Build history of the part. All positions in model axes, mm. Face numbers are marked on the shaded views. A direction names the side the tool comes from. Give positions to 0.01 mm unless a question says otherwise; leave off trailing zeros. Loops run counter-clockwise (first coordinate to the right, second up) from the corner with the lowest first, then second, coordinate; pieces in that order, holes last. Notation, with made-up numbers: (58, 70) -> (83, 70) arc R24 ccw to (83, 95) -> close; hole circle Ø1 at (6, -1). An arc over 180 degrees is marked (long way). One line per question, with ' | ' between items. Start each with the question number.
(1) 3-axis set-ups, long thin cutter, end or side, ignore diameter. For the marked faces 5, 6, 7 and 8: which of +Z, -Z, +X, -X, +Y, -Y reach the whole face in a straight line?
(2) Slice it at C-C, the plane z = 27. Write the cut outline in (x, y), then the cut area to 3 significant figures.
(3) Mould opens along X. For the marked faces 1, 2, 3 and 4 say: pulls with the +X half, pulls with the -X half, needs draft (parallel to the pull), parting line crosses it, or undercut.
(4) Slice it at A-A, the plane x = 26. Write the cut outline in (y, z), then the cut area to 3 significant figures.
(5) Slice it at B-B, the plane y = 44.5. Write the cut outline in (x, z), then the cut area to 3 significant figures.
(6) Slice it at D-D, the plane z = 14. Write the cut outline in (x, y), then the cut area to 3 significant figures.
(7) Flat gauge pins, fed straight in: pin 1 Ø2.5 at (x, z) = (25, 13.5) entering from -Y; pin 2 Ø1.6 at (x, z) = (14, 16) entering from -Y; pin 3 Ø13 at (x, z) = (36, 28) entering from +Y; pin 4 Ø1 at (x, y) = (10.5, 16.5) entering from +Z. Where does each tip first touch, or does it go through?
(8) Drill centre lines: L1, parallel to Y at x = 9, z = 13.25; L2, parallel to Y at x = 10.5, z = 14.75; L3, parallel to Y at x = 25, z = 25.5. Where is each one in solid material? Low to high. Write a range as from..to.
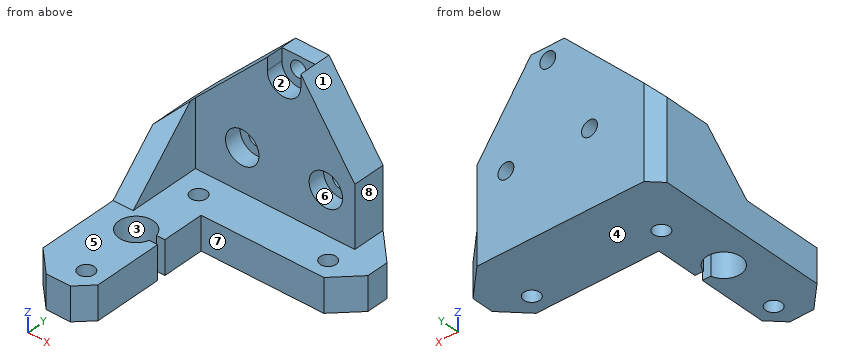
```python
from build123d import *

# Parameters (mm, degrees)
SKETCH_R        = 1.9
SKETCH_R_2      = 4.1
PAD_DEPTH       = 8
PAD001_DEPTH    = 33
SKETCH002_R     = 1.9
POCKET_DEPTH    = 7.801
POCKET001_DEPTH = 5
POCKET002_DEPTH = 50.001
CHAMFER_SIZE    = 3
SKETCH005_R     = 4
POCKET003_DEPTH = 4
SKETCH006_W     = 2.5
SKETCH006_H     = 2
POCKET004_DEPTH = 8.001


with BuildPart() as part:
    # Sketch → Pad (new body)
    with BuildSketch(Plane.XY.offset(10)):
        Polygon((0, 50), (0, 5.656854), (5.656854, 0), (11.464466, 0), (15, 3.535534), (15, 32), (44.343146, 32), (50, 37.656854), (50, 42.928932), (42.928932, 50), align=None)
        with Locations((41.5, 36.5)):
            Circle(SKETCH_R, mode=Mode.SUBTRACT)
        with Locations((10.5, 36.5)):
            Circle(SKETCH_R, mode=Mode.SUBTRACT)
        with Locations((10.5, 5.5)):
            Circle(SKETCH_R, mode=Mode.SUBTRACT)
        with Locations((9, 21)):
            Circle(SKETCH_R_2, mode=Mode.SUBTRACT)
    extrude(amount=PAD_DEPTH)

    # Sketch001 → Pad001 (new body)
    with BuildSketch(Plane.XY.offset(18)):
        Polygon((42.928932, 50), (0, 50), (0, 25), (4.8, 25), (4.8, 42.2), (42.928932, 42.2), align=None)
    extrude(amount=PAD001_DEPTH)

    # Sketch002 → Pocket (cut, through all)
    with BuildSketch(Plane(origin=(0, 42.2, 10), x_dir=(1, 0, 0), z_dir=(0, -1, 0))):
        with Locations((26, 38)):
            Circle(SKETCH002_R)
        with Locations((16, 18)):
            Circle(SKETCH002_R)
        with Locations((36, 18)):
            Circle(SKETCH002_R)
    extrude(amount=-POCKET_DEPTH, mode=Mode.SUBTRACT)

    # Sketch003 → Pocket001 (cut)
    with BuildSketch(Plane(origin=(4.8, 0, 10), x_dir=(0, 1, 0), z_dir=(1, 0, 0))):
        Polygon((25, 8), (42.2, 25.2), (42.2, 41), (25, 41), align=None)
    extrude(amount=-POCKET001_DEPTH, mode=Mode.SUBTRACT)

    # Sketch004 → Pocket002 (cut, through all)
    with BuildSketch(Plane(origin=(0, 50, 10), x_dir=(-1, 0, 0), z_dir=(0, 1, 0))):
        Polygon((-42.928932, 22.535571), (-30, 41), (-42.928932, 41), align=None)
        Polygon((-22, 41), (0, 19), (0, 41), align=None)
    extrude(amount=-POCKET002_DEPTH, mode=Mode.SUBTRACT)

    # Chamfer
    chamfer_edges = [part.edges().sort_by_distance(p)[0] for p in [
        (0, 50, 23.5),
    ]]
    chamfer(chamfer_edges, length=CHAMFER_SIZE)

    # Sketch005 → Pocket003 (cut)
    with BuildSketch(Plane(origin=(0, 42.2, 10), x_dir=(1, 0, 0), z_dir=(0, -1, 0))):
        with Locations((16, 18)):
            Circle(SKETCH005_R)
        with Locations((36, 18)):
            Circle(SKETCH005_R)
        with BuildLine():
            ThreePointArc((22, 37.999999), (26, 34), (30, 37.999999))
            Line((30, 37.999999), (30, 41))
            Line((22, 41), (30, 41))
            Line((22, 37.999999), (22, 41))
        make_face()
    extrude(amount=-POCKET003_DEPTH, mode=Mode.SUBTRACT)

    # Sketch006 → Pocket004 (cut, through all)
    with BuildSketch(Plane.XY.offset(18)):
        with Locations((13.75, 21)):
            Rectangle(SKETCH006_W, SKETCH006_H)
    extrude(amount=-POCKET004_DEPTH, mode=Mode.SUBTRACT)


solid = part.part
```
Final values:
1) face 5: +Z, +X, -Y | face 6: -Y | face 7: +Z, -Z, +X, -Y | face 8: +Z, +X, +Y, -Y
2) outline: (0, 34) -> (4.8, 34) -> (4.8, 42.2) -> (12.13, 42.2) -> (12.13, 46.2) -> (14.38, 46.2) -> (14.38, 50) -> (3, 50) -> (0, 47) -> close; (17.62, 46.2) -> (19.87, 46.2) -> (19.87, 42.2) -> (32.13, 42.2) -> (32.13, 46.2) -> (34.38, 46.2) -> (34.38, 50) -> (17.62, 50) -> close; (37.62, 46.2) -> (39.87, 46.2) -> (39.87, 42.2) -> (42.93, 42.2) -> (42.93, 50) -> (37.62, 50) -> close | area: 283 mm2
3) face 1: pulls with the +X half | face 2: undercut | face 3: undercut | face 4: needs draft
4) outline: (32, 10) -> (50, 10) -> (50, 46.1) -> (46.2, 46.1) -> (46.2, 44) -> (42.2, 44) -> (42.2, 18) -> (32, 18) -> close; (46.2, 49.9) -> (50, 49.9) -> (50, 51) -> (46.2, 51) -> close | area: 359 mm2
5) outline: (0, 10) -> (48.43, 10) -> (48.43, 18) -> (42.93, 18) -> (42.93, 32.54) -> (30, 51) -> (30, 48) arc R4 cw to (22, 48) -> (22, 51) -> (0, 29) -> close; hole circle Ø8 at (16, 28); hole circle Ø8 at (36, 28) | area: 1,290 mm2
6) outline: (0, 5.66) -> (5.66, 0) -> (11.46, 0) -> (15, 3.54) -> (15, 20) -> (12.98, 20) arc R4.1 cw (long way) to (12.98, 22) -> (15, 22) -> (15, 32) -> (44.34, 32) -> (50, 37.66) -> (50, 42.93) -> (42.93, 50) -> (3, 50) -> (0, 47) -> close; hole circle Ø3.8 at (10.5, 5.5); hole circle Ø3.8 at (10.5, 36.5); hole circle Ø3.8 at (41.5, 36.5) | area: 1,220 mm2
7) pin 1: y = 32 | pin 2: y = 1.74 | pin 3: y = 50 | pin 4: z = 18
8) L1: 0..4.33, 6.67..16.9, 25.1..35.33, 37.67..50 | L2: 0..3.6, 7.4..17.18, 24.82..34.6, 38.4..50 | L3: 42.2..50
